from build123d import *

# Parameters (mm, degrees)
F0_W      = 64.5
F0_H      = 101.3
F1_DEPTH  = 3
F1_FACE_W = 64.5
F1_FACE_H = 101.3
F2_DEPTH  = 11
F3_W      = 60.5
F3_H      = 97.3
F4_DEPTH  = 11


with BuildPart() as f1:
    # F0 (on Top) → F1 (new body)
    with BuildSketch(Plane.XY):
        with Locations((32.25, 50.65)):
            Rectangle(F0_W, F0_H)
    extrude(amount=F1_DEPTH)

    # F1_face (on face) → F2 (join)
    with BuildSketch(Plane(origin=(32.25, 50.65, 3), x_dir=(1, 0, 0), z_dir=(0, 0, 1))):
        Rectangle(F1_FACE_W, F1_FACE_H)
    extrude(amount=F2_DEPTH)

    # F3 (on face) → F4 (cut)
    with BuildSketch(Plane.XY.offset(14)):
        with Locations((32.25, 50.65)):
            Rectangle(F3_W, F3_H)
    extrude(amount=-F4_DEPTH, mode=Mode.SUBTRACT)


solid = f1.part
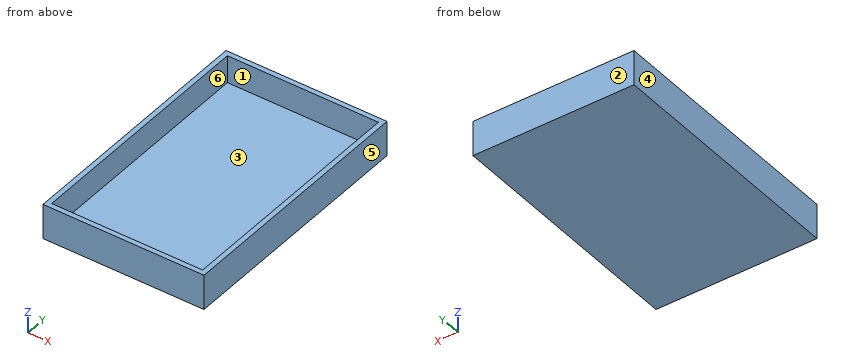
Source: CAD feature listing. Evaluate the final solid. Frame: model axes, mm. Face numbers are marked on the shaded views. A direction names the side the tool comes from. Round coordinates to 2 decimals unless told otherwise and drop trailing zeros. Loops run counter-clockwise (first coordinate to the right, second up) from the corner with the lowest first, then second, coordinate; pieces in that order, holes last. Notation, with made-up numbers: M 29,89.5 L 47,89.5 A23 cw 47,102.5 Z; hole C -2,49 d8. An arc over 180 degrees is marked long. Return JSON: item names as keys, results as strings. Group by question number.
1. Reachability of the marked faces 1 and 2 from +Z, -Z, +X, -X, +Y, -Y: full face, straight path, thin tool, end or side. Return the list, or none.
2. Section query A-A on z = 11. Output: boundary loops of the cut face in (x, y), and give its area (3 significant figures).
3. Material intervals for line 1 along Y through (x, z) = (6, 10.25); line 2 along X through (y, z) = (54.5, 12.5); line 3 along Z through (x, y) = (24, 45), sorted ascending. Write a range as from..to.
4. Pin query (flat end, axial travel): pin 1 (1.5 mm diameter, centred on x = 16, y = 24.5, fed in from +Z). Return the tip coordinate at first contact, or that it passes through.
5. Section query B-B on y = 18. Output: boundary loops of the cut face in (x, z).
6. Mould query, pull axis X, two halves, no side actions, for the marked faces 3, 4, 5 and 6. Classes: released by +X, released by -X, zero draft, split by the parting line, or undercut.
7. Section query C-C on x = 17. Output: boundary loops of the cut face in (y, z).
Checks:
{
 "1": {"face 1": "+Z", "face 2": "+Z, -Z, +X, -X, +Y"},
 "2": {"outline": "M 0,0 L 64.5,0 L 64.5,101.3 L 0,101.3 Z; hole M 2,2 L 62.5,2 L 62.5,99.3 L 2,99.3 Z", "area": "647 mm²"},
 "3": {"line 1": "y = 0..2, 99.3..101.3", "line 2": "x = 0..2, 62.5..64.5", "line 3": "z = 0..3"},
 "4": {"pin 1": "stops at z = 3"},
 "5": {"outline": "M 0,0 L 64.5,0 L 64.5,14 L 62.5,14 L 62.5,3 L 2,3 L 2,14 L 0,14 Z"},
 "6": {"face 3": "undercut", "face 4": "released by -X", "face 5": "released by +X", "face 6": "undercut"},
 "7": {"outline": "M 0,0 L 101.3,0 L 101.3,14 L 99.3,14 L 99.3,3 L 2,3 L 2,14 L 0,14 Z"}
}
